CAD build for the part. Positions are in the model's coordinates, mm. A direction names the side the tool comes from. Coordinates: 2 decimals unless noted, no trailing zeros. Order: outer loops, then holes, each group sorted by start corner. A loop starts at its lowest first (then second) coordinate and runs counter-clockwise, first axis right, second up. Notation, with made-up numbers: (60.5, 18) - (69.5, 18) arc R29 ccw to (69.5, 39) - close; hole circle Ø2 at (41.25, 25). An arc over 180 degrees is marked (long way). Write each question's results on one line, items separated by ' | '. Start each with the question number.
Q1. Band-saw the part on C-C, the plane x = -10.5. Write the cut outline in (y, z), then the cut area to 3 significant figures.
Q2. Band-saw the part on D-D, the plane z = -5.5. Write the cut outline in (x, y), then the cut area to 3 significant figures.
Q3. Pull direction Z, two halves, no side cores. Call faces 1 (the flat face through (0, 0, 0)), 2 (the flat face through (21, 0, -2)), 3 (the cylindrical face through (19.77, 3.38, -4.19)): released by +Z, released by -Z, zero draft, split by the parting line, or undercut.
Q4. Band-saw the part on A-A, the plane y = 3. Write the cut outline in (x, z), then the cut area to 4 significant figures.
Q5. Which spindle directions (+Z, -Z, +X, -X, +Y, -Y) get a long thin tool onto all of the face, cutting with end or side? Do faces 4 (the flat face through (0, 5, -2)), 5 (the cylindrical face through (-19.73, 3.38, -4.19)), 6 (the flat face through (0, -6, -3)). Say none if no direction does.
Q6. Wall check: probe 1 along Y at (x, z) = (19.5, -3); probe 2 along X at (y, z) = (1.5, -1.25); probe 3 along Y at (x, z) = (-1, -1.25). Give the ranges that are in metal, low to high.
Q7. Band-saw the part on B-B, the plane z = -2.25. Write the cut outline in (x, y).
Q8. Pin check, flat tips, straight feed: P1, Ø2, axis at y = 3, z = -3, coming from the +X side; P2, Ø2, axis at x = 2, y = 6.5, coming from the -Z side. Stop position of each tip, or through.
```python
from build123d import *

# Parameters (mm, degrees)
SKETCH1_W           = 42
SKETCH1_H           = 14
BOSS_EXTRUDE1_DEPTH = 2
SKETCH2_W           = 2.5
SKETCH2_H           = 14
BOSS_EXTRUDE2_DEPTH = 6
SKETCH5_R           = 1.25
CUT_EXTRUDE1_DEPTH  = 43
BOSS_EXTRUDE3_DEPTH = 2


with BuildPart() as part:
    # Sketch1 → Boss-Extrude1 (new body)
    with BuildSketch(Plane.XY):
        Rectangle(SKETCH1_W, SKETCH1_H)
    extrude(amount=BOSS_EXTRUDE1_DEPTH)

    # Sketch2 → Boss-Extrude2 (add)
    with BuildSketch(Plane(origin=(0, 0, 0), x_dir=(-1, 0, 0), z_dir=(0, 0, -1))):
        with Locations((-19.75, 0)):
            Rectangle(SKETCH2_W, SKETCH2_H)
        with Locations((19.75, 0)):
            Rectangle(SKETCH2_W, SKETCH2_H)
    extrude(amount=BOSS_EXTRUDE2_DEPTH)

    # Sketch5 → Cut-Extrude1 (cut, through all)
    with BuildSketch(Plane(origin=(21, 0, 0), x_dir=(0, 0, -1), z_dir=(1, 0, 0))):
        with Locations((3, 3)):
            Circle(SKETCH5_R)
        with Locations((3, -3)):
            Circle(SKETCH5_R)
    extrude(amount=-CUT_EXTRUDE1_DEPTH, mode=Mode.SUBTRACT)

    # Sketch6 → Boss-Extrude3 (add)
    with BuildSketch(Plane(origin=(0, 7, 0), x_dir=(1, 0, 0), z_dir=(0, 1, 0))):
        Polygon((-18.5, 6), (-18.5, 0), (-12.5, 0), (12.5, 0), (18.5, 0), (18.5, 6), (15.5, 3), (-15.5, 3), align=None)
    boss_extrude3 = extrude(amount=-BOSS_EXTRUDE3_DEPTH)

    # Mirror1: Boss-Extrude3 across plane
    add(boss_extrude3.mirror(Plane.ZX))


solid = part.part
```
Results below:
1) outline: (-7, -3) - (-5, -3) - (-5, 0) - (5, 0) - (5, -3) - (7, -3) - (7, 2) - (-7, 2) - close | area: 40.0 mm²
2) outline: (-21, -7) - (-18, -7) - (-18, -5) - (-18.5, -5) - (-18.5, 5) - (-18, 5) - (-18, 7) - (-21, 7) - close; (18, -7) - (21, -7) - (21, 7) - (18, 7) - (18, 5) - (18.5, 5) - (18.5, -5) - (18, -5) - close | area: 74.0 mm²
3) face 1: released by -Z | face 2: zero draft | face 3: undercut
4) outline: (-21, -6) - (-18.5, -6) - (-18.5, -4.25) - (-21, -4.25) - close; (-21, -1.75) - (-18.5, -1.75) - (-18.5, 0) - (18.5, 0) - (18.5, -1.75) - (21, -1.75) - (21, 2) - (-21, 2) - close; (18.5, -6) - (21, -6) - (21, -4.25) - (18.5, -4.25) - close | area: 101.5 mm²
5) face 4: -Z | face 5: +X, -X | face 6: -Z, +Y, -Y
6) probe 1: y = -7 to -4.25, -1.75 to 1.75, 4.25 to 7 | probe 2: x = -21 to -18.5, 18.5 to 21 | probe 3: y = -7 to -5, 5 to 7
7) outline: (-21, -7) - (21, -7) - (21, -4) - (18.5, -4) - (18.5, -5) - (-18.5, -5) - (-18.5, -4) - (-21, -4) - close; (-21, -2) - (-18.5, -2) - (-18.5, 2) - (-21, 2) - close; (-21, 4) - (-18.5, 4) - (-18.5, 5) - (18.5, 5) - (18.5, 4) - (21, 4) - (21, 7) - (-21, 7) - close; (18.5, -2) - (21, -2) - (21, 2) - (18.5, 2) - close
8) P1: passes through | P2: stops at z = -3
